from build123d import *

# Parameters (mm, degrees)
SKETCH1_W           = 22
SKETCH1_H           = 13
BOSS_EXTRUDE1_DEPTH = 6
BOSS_EXTRUDE2_DEPTH = 3.5
BOSS_EXTRUDE3_DEPTH = 9.5
SKETCH4_R           = 1.525
SKETCH4_R_2         = 1.524
CUT_EXTRUDE1_DEPTH  = 36.933967218
SKETCH5_W           = 9
SKETCH5_H           = 5.5
CUT_EXTRUDE2_DEPTH  = 39.082148049
FILLET1_R           = 2
SKETCH6_W           = 12
SKETCH6_H           = 13.009000019
SKETCH6_W_2         = 15.838286437
CUT_EXTRUDE3_DEPTH  = 4
BOSS_EXTRUDE4_DEPTH = 23
CUT_EXTRUDE4_DEPTH  = 23
SKETCH9_R           = 4.9
CUT_EXTRUDE6_DEPTH  = 23
SKETCH10_R          = 1.5
CUT_EXTRUDE7_DEPTH  = 23
BOSS_EXTRUDE5_DEPTH = 3
FILLET2_R           = 2.5
FILLET3_R           = 2.5
SKETCH12_W          = 20
SKETCH12_H          = 3
CUT_EXTRUDE8_DEPTH  = 1.5
BOSS_EXTRUDE6_DEPTH = 8
SKETCH15_R          = 4.9
SKETCH15_R_2        = 1.5
CUT_EXTRUDE9_DEPTH  = 48.51052515
SKETCH16_W          = 29.561254557
SKETCH16_H          = 40.782628596
CUT_EXTRUDE10_DEPTH = 3
SKETCH17_W          = 8
SKETCH17_H          = 5.5
BOSS_EXTRUDE7_DEPTH = 9.5
CUT_EXTRUDE11_DEPTH = 1.5
SKETCH20_R          = 2.5
CUT_EXTRUDE12_DEPTH = 2.5
SKETCH19_W          = 3.25
SKETCH19_H          = 19
CUT_EXTRUDE13_DEPTH = 1
CHAMFER1_SIZE       = 1
FILLET4_R           = 3


with BuildPart() as part:
    # Sketch1 → Boss-Extrude1 (new body)
    with BuildSketch(Plane(origin=(0, 0, 0), x_dir=(1, 0, 0), z_dir=(0, 1, 0))):
        with BuildLine():
            Line((-1, -3), (23, -3))
            Line((23, -3), (25, -3))
            Line((25, -3), (25, -1))
            Line((25, -1), (25, 14))
            Line((25, 14), (25, 16))
            Line((25, 16), (23, 16))
            Line((23, 16), (-1, 16))
            ThreePointArc((-1, 16), (-2.414213562, 15.414213562), (-3, 14))
            Line((-3, 14), (-3, -1))
            ThreePointArc((-3, -1), (-2.414213562, -2.414213562), (-1, -3))
        make_face()
        with Locations((11, 6.5)):
            Rectangle(SKETCH1_W, SKETCH1_H, mode=Mode.SUBTRACT)
    extrude(amount=BOSS_EXTRUDE1_DEPTH)

    # Sketch2 → Boss-Extrude2 (add)
    with BuildSketch(Plane(origin=(0, 6, 0), x_dir=(1, 0, 0), z_dir=(0, 1, 0))):
        with BuildLine():
            Line((25, 14), (25, -1))
            Line((25, -1), (25, -3))
            Line((25, -3), (23, -3))
            Line((23, -3), (-1, -3))
            ThreePointArc((-1, -3), (-2.414213562, -2.414213562), (-3, -1))
            Line((-3, -1), (-3, 14))
            ThreePointArc((-3, 14), (-2.414213562, 15.414213562), (-1, 16))
            Line((-1, 16), (23, 16))
            Line((23, 16), (25, 16))
            Line((25, 16), (25, 14))
        make_face()
    extrude(amount=BOSS_EXTRUDE2_DEPTH)

    # Sketch3 → Boss-Extrude3 (add)
    with BuildSketch(Plane.XZ):
        with BuildLine():
            Line((5, 3), (17, 3))
            Line((17, 3), (17, 5.5))
            ThreePointArc((17, 5.5), (15.389087297, 9.389087297), (11.5, 11))
            Line((11.5, 11), (10.5, 11))
            ThreePointArc((10.5, 11), (6.610912703, 9.389087297), (5, 5.5))
            Line((5, 5.5), (5, 3))
        make_face()
        with BuildLine():
            Line((17, -16), (5, -16))
            Line((5, -16), (5, -18.5))
            ThreePointArc((5, -18.5), (6.610912703, -22.389087297), (10.5, -24))
            Line((10.5, -24), (11.5, -24))
            ThreePointArc((11.5, -24), (15.389087297, -22.389087297), (17, -18.5))
            Line((17, -18.5), (17, -16))
        make_face()
    extrude(amount=-BOSS_EXTRUDE3_DEPTH)

    # Sketch4 → Cut-Extrude1 (cut, through all)
    with BuildSketch(Plane(origin=(0, 0, 0), x_dir=(-1, 0, 0), z_dir=(0, -1, 0))):
        with Locations(Location((-11, 20, 0), (0, 0, 90))):
            Circle(SKETCH4_R)
        with Locations(Location((-11, -7, 0), (0, 0, 90))):
            Circle(SKETCH4_R_2)
    extrude(amount=-CUT_EXTRUDE1_DEPTH, mode=Mode.SUBTRACT)

    # Sketch5 → Cut-Extrude2 (cut, through all)
    with BuildSketch(Plane(origin=(25, 0, 0), x_dir=(0, 0, -1), z_dir=(1, 0, 0))):
        with Locations((6.5, 2.75)):
            Rectangle(SKETCH5_W, SKETCH5_H)
    extrude(amount=-CUT_EXTRUDE2_DEPTH, mode=Mode.SUBTRACT)

    # Fillet1
    fillet1_edges = [part.edges().sort_by_distance(p)[0] for p in [
        (-1.5, 5.5, -11),
        (-1.5, 5.5, -2),
        (23.5, 5.5, -11),
        (23.5, 5.5, -2),
    ]]
    fillet(fillet1_edges, radius=FILLET1_R)

    # Sketch6 → Cut-Extrude3 (cut)
    with BuildSketch(Plane(origin=(0, 9.5, 0), x_dir=(1, 0, 0), z_dir=(0, 1, 0))):
        with Locations((11, 22.504500009)):
            Rectangle(SKETCH6_W, SKETCH6_H)
        with Locations((11.149066226, -9.50450001)):
            Rectangle(SKETCH6_W_2, SKETCH6_H)
    extrude(amount=-CUT_EXTRUDE3_DEPTH, mode=Mode.SUBTRACT)

    # Sketch7 → Boss-Extrude4 (add)
    with BuildSketch(Plane(origin=(0, 9.5, 0), x_dir=(1, 0, 0), z_dir=(0, 1, 0))):
        Polygon((23, 16), (22, 16), (22, -3), (23, -3), (25, -3), (25, -1), (25, 14), (25, 16), align=None)
    extrude(amount=BOSS_EXTRUDE4_DEPTH)

    # Sketch8 → Cut-Extrude4 (cut)
    with BuildSketch(Plane(origin=(0, 9.5, 0), x_dir=(1, 0, 0), z_dir=(0, 1, 0))):
        with BuildLine():
            Line((-3, 2), (0, 2))
            ThreePointArc((0, 2), (1.414213562, 2.585786438), (2, 4))
            Line((2, 4), (2, 9))
            ThreePointArc((2, 9), (1.414213562, 10.414213562), (0, 11))
            Line((0, 11), (-3, 11))
            Line((-3, 11), (-3, 2))
        make_face()
    extrude(amount=-CUT_EXTRUDE4_DEPTH, mode=Mode.SUBTRACT)

    # Sketch9 → Cut-Extrude6 (cut)
    with BuildSketch(Plane.ZY.offset(-22)):
        with Locations((-6.5, 17.5)):
            Circle(SKETCH9_R)
    extrude(amount=-CUT_EXTRUDE6_DEPTH, mode=Mode.SUBTRACT)

    # Sketch10 → Cut-Extrude7 (cut)
    with BuildSketch(Plane.ZY.offset(-22)):
        with Locations((-12, 11.5)):
            Circle(SKETCH10_R)
        with Locations((-1, 11.5)):
            Circle(SKETCH10_R)
    extrude(amount=-CUT_EXTRUDE7_DEPTH, mode=Mode.SUBTRACT)

    # Sketch11 → Boss-Extrude5 (add)
    with BuildSketch(Plane(origin=(25, 0, 0), x_dir=(0, 0, -1), z_dir=(1, 0, 0))):
        with BuildLine():
            Line((-3, 0), (-5.5, 0))
            Line((-5.5, 0), (-5.5, 11.617902622))
            ThreePointArc((-5.5, 11.617902622), (-4.914213562, 13.032116185), (-3.5, 13.617902622))
            Line((-3.5, 13.617902622), (-3, 13.617902622))
            Line((-3, 13.617902622), (-3, 0))
        make_face()
        with BuildLine():
            Line((16, 0), (18.5, 0))
            Line((18.5, 0), (18.5, 11.617902622))
            ThreePointArc((18.5, 11.617902622), (17.914213562, 13.032116185), (16.5, 13.617902622))
            Line((16.5, 13.617902622), (16, 13.617902622))
            Line((16, 13.617902622), (16, 0))
        make_face()
    extrude(amount=-BOSS_EXTRUDE5_DEPTH)

    # Fillet2
    fillet2_edges = [part.edges().sort_by_distance(p)[0] for p in [
        (22, 4.75, 3),
    ]]
    fillet(fillet2_edges, radius=FILLET2_R - 0.0001)  # a hair under: the kernel refuses the full size

    # Fillet3
    fillet3_edges = [part.edges().sort_by_distance(p)[0] for p in [
        (22, 4.75, -16),
    ]]
    fillet(fillet3_edges, radius=FILLET3_R - 0.0001)  # a hair under: the kernel refuses the full size

    # Sketch12 → Cut-Extrude8 (cut)
    with BuildSketch(Plane.XZ.offset(-6)):
        with Locations((12, -6.5)):
            Rectangle(SKETCH12_W, SKETCH12_H)
    extrude(amount=-CUT_EXTRUDE8_DEPTH, mode=Mode.SUBTRACT)

    # Sketch14 → Boss-Extrude6 (add)
    with BuildSketch(Plane.ZY.offset(-22)):
        with BuildLine():
            Line((-16, 32.5), (3, 32.5))
            Line((3, 32.5), (3, 13.617902622))
            ThreePointArc((3, 13.617902622), (4.730624847, 13.218683682), (5.5, 11.617902622))
            Line((5.5, 11.617902622), (5.5, 9.5))
            Line((5.5, 9.5), (3, 9.5))
            Line((3, 9.5), (-16, 9.5))
            Line((-16, 9.5), (-18.5, 9.5))
            Line((-18.5, 9.5), (-18.5, 11.617902622))
            ThreePointArc((-18.5, 11.617902622), (-17.730624847, 13.218683682), (-16, 13.617902622))
            Line((-16, 13.617902622), (-16, 32.5))
        make_face()
    extrude(amount=BOSS_EXTRUDE6_DEPTH)

    # Sketch15 → Cut-Extrude9 (cut, through all)
    with BuildSketch(Plane(origin=(22, 0, 0), x_dir=(0, 0, -1), z_dir=(1, 0, 0))):
        with Locations(Location((6.5, 17.5, 0), (0, 0, 180))):
            Circle(SKETCH15_R)
        with Locations(Location((1, 11.5, 0), (0, 0, 180))):
            Circle(SKETCH15_R_2)
        with Locations(Location((12, 11.5, 0), (0, 0, 180))):
            Circle(SKETCH15_R_2)
    extrude(amount=-CUT_EXTRUDE9_DEPTH, mode=Mode.SUBTRACT)

    # Sketch16 → Cut-Extrude10 (cut)
    with BuildSketch(Plane(origin=(25, 0, 0), x_dir=(0, 0, -1), z_dir=(1, 0, 0))):
        with Locations((4.352462689, 15.924842514)):
            Rectangle(SKETCH16_W, SKETCH16_H)
    extrude(amount=-CUT_EXTRUDE10_DEPTH, mode=Mode.SUBTRACT)

    # Sketch17 → Boss-Extrude7 (add)
    with BuildSketch(Plane.XZ):
        with Locations((18, -15.75)):
            Rectangle(SKETCH17_W, SKETCH17_H)
        with Locations((18, 2.75)):
            Rectangle(SKETCH17_W, SKETCH17_H)
    extrude(amount=-BOSS_EXTRUDE7_DEPTH)

    # Sketch18 → Cut-Extrude11 (cut)
    with BuildSketch(Plane(origin=(0, 6, 0), x_dir=(-1, 0, 0), z_dir=(0, -1, 0))):
        Polygon((-22, 2.5), (-17, 5), (-17, 8), (-22, 10.5), align=None)
    extrude(amount=-CUT_EXTRUDE11_DEPTH, mode=Mode.SUBTRACT)

    # Sketch20 → Cut-Extrude12 (cut)
    with BuildSketch(Plane(origin=(22, 0, 0), x_dir=(0, 0, -1), z_dir=(1, 0, 0))):
        with Locations((1, 11.5)):
            Circle(SKETCH20_R)
        with Locations((12, 11.5)):
            Circle(SKETCH20_R)
    extrude(amount=-CUT_EXTRUDE12_DEPTH, mode=Mode.SUBTRACT)

    # Sketch19 → Cut-Extrude13 (cut)
    with BuildSketch(Plane(origin=(0, 9.5, 0), x_dir=(1, 0, 0), z_dir=(0, 1, 0))):
        with Locations((12.375, 6.5)):
            Rectangle(SKETCH19_W, SKETCH19_H)
    extrude(amount=-CUT_EXTRUDE13_DEPTH, mode=Mode.SUBTRACT)

    # Chamfer1
    chamfer1_edges = [part.edges().sort_by_distance(p)[0] for p in [
        (14, 17.5, -11.4),
    ]]
    chamfer(chamfer1_edges, length=CHAMFER1_SIZE)

    # Fillet4
    fillet4_edges = [part.edges().sort_by_distance(p)[0] for p in [
        (18, 32.5, 3),
        (18, 32.5, -16),
    ]]
    fillet(fillet4_edges, radius=FILLET4_R)


solid = part.part
Verification items for the finished model (mm, model axes). A direction names the side the tool comes from. Coordinates: 2 decimals unless noted, no trailing zeros. Order: outer loops, then holes, each group sorted by start corner. A loop starts at its lowest first (then second) coordinate and runs counter-clockwise, first axis right, second up. Notation, with made-up numbers: M 36.25,1.25 L 78.25,1.25 A16 ccw 78.25,16.25 Z; hole C -18,16 d9. An arc over 180 degrees is marked long. One line per item, written item: value. Start each with the question number.
Item 1: Sectioned sample at C-C (z = -20). Enter the section's corners in (x, y) (1 decimal).
Item 2: Scan lines: probe 1 along Z at (x, y) = (16.5, 17.5); probe 2 along Z at (x, y) = (16.3, 11.5); probe 3 along Y at (x, z) = (15.65, -12). Record each from-to range of solid material in increasing order.
Item 3: Sectioned sample at D-D (x = 2.5). Enter the section's corners in (y, z), then the cut area to 3 significant figures.
Item 4: Sectioned sample at B-B (y = 17.5). Enter the section's corners in (x, z), then the cut area to 3 significant figures.
Item 5: Mould release check, pull along Y, two halves, no side actions. Record for faces 4 (the flat face through (14, 7.5, -7)), 5 (the cylindrical face through (15.35, 2.71, -22.43)), 6 (the flat face through (5, 9.5, -7)), 7 (the flat face through (19.5, 10, -13)): released by +Y, released by -Y, zero draft, split by the parting line, or undercut.
Item 6: Access from +Z, -Z, +X, -X, +Y, -Y to the whole of each face (thin tool, end or side, straight path). Record for faces 1 (the flat face through (10.75, 9, -6)), 2 (the flat face through (11, 6, -3)), 3 (the flat face through (-1, 5, -11)).
Item 7: Gauge pin test, flat ends, axial feed: pin 1 (6 mm diameter, centred on x = 8.5, z = -5, fed in from +Y); pin 2 (6.5 mm diameter, centred on x = 16.5, y = 4.5, fed in from +Z); pin 3 (8 mm diameter, centred on x = 15, y = 26, fed in from +Z); pin 4 (4 mm diameter, centred on y = 5, z = 2.5, fed in from -X). Record the tip position at first contact, or that the pin passes through.
Item 8: Sectioned sample at A-A (y = 4.5). Enter the section's corners in (x, z) (3 decimals), then the cut area to 3 significant figures.
Conclusion:
1. outline: M 5.2,0 L 9.5,0 L 9.5,5.5 L 5.2,5.5 Z; M 12.5,0 L 16.8,0 L 16.8,5.5 L 12.5,5.5 Z
2. probe 1: z = -16 to -11.4, -1.6 to 3
2. probe 2: z = -18.5 to -13.5, -10.5 to -2.5, 0.5 to 5.5
2. probe 3: y = 6 to 10, 13 to 32.5
3. outline: M 0,-16 L 9.5,-16 L 9.5,3 L 0,3 L 0,0 L 6,0 L 6,-5 L 7.5,-5 L 7.5,-8 L 6,-8 L 6,-13 L 0,-13 Z
3. area: 98.0 mm^2
4. outline: M 14,-16 L 22,-16 L 22,-11.4 L 15,-11.4 L 14,-12.4 Z; M 14,-0.6 L 15,-1.6 L 22,-1.6 L 22,3 L 14,3 Z
4. area: 72.6 mm^2
5. face 4: released by -Y
5. face 5: zero draft
5. face 6: released by +Y
5. face 7: undercut
6. face 1: +Z, -Z, +Y
6. face 2: +X, -Y
6. face 3: -X, +Y, -Y
7. pin 1: stops at y = 9.5
7. pin 2: stops at z = 10.71
7. pin 3: stops at z = 3
7. pin 4: stops at x = -3
8. outline: M -3,-14 A2 ccw -1,-16 L 5,-16 L 5,-18.5 A5.5 ccw 10.5,-24 L 11.5,-24 A5.5 ccw 17,-18.5 L 22,-18.5 L 22,-13 L 0,-13 L 0,-11 L -3,-11 Z; M -3,-2 L 0,-2 L 0,0 L 22,0 L 22,5.5 L 17,5.5 A5.5 ccw 11.5,11 L 10.5,11 A5.5 ccw 5,5.5 L 5,3 L -1,3 A2 ccw -3,1 Z; hole C 11,-20 d3.05; hole C 11,7 d3.048
8. area: 337 mm^2
